The model under review builds one solid part; all positions refer to its coordinate system, in mm. Face numbers are marked on the shaded views. A direction names the side the tool comes from. Give positions to 0.01 mm unless a question says otherwise; leave off trailing zeros. Loops run counter-clockwise (first coordinate to the right, second up) from the corner with the lowest first, then second, coordinate; pieces in that order, holes last. Notation, with made-up numbers: M -6,71 L 43,71 A17 ccw 43,78 Z; hole C 76,73 d5. An arc over 180 degrees is marked long. One line per item, written item: value. Start each with the question number.
Q1. To check wall thickness, follow line 1 along X through (y, z) = (1.75, 0.5); line 2 along X through (y, z) = (1.5, 3.45); line 3 along Y through (x, z) = (-7.75, 3.6). State the ranges of each line that lie inside material, in increasing order. Write a range as from..to.
Q2. We need section A-A on y = 0. Write out the cut boundary in (x, z), plus the area to 3 significant figures.
Q3. For the marked faces 5, 6, 7, 8 and 9, list the 3-axis set-ups (+Z, -Z, +X, -X, +Y, -Y) from which the entire face can be reached by the end or side of a thin tool; tool diameter is ignored.
Q4. We need section C-C on y = 10. Write out the cut boundary in (x, z), plus the area to 3 significant figures.
Q5. Mouldability with a two-part tool opening along Y and no side actions: class the marked faces 1, 2, 3 and 4 as released by +Y, released by -Y, zero draft, split by the parting line, or undercut.
Q6. We need section B-B on x = 8.5. Write out the cut boundary in (y, z), plus the area to 3 significant figures.
Q7. For pin 1 (1.5 mm diameter, centred on x = -6, y = -8.5, fed in from +Z); pin 2 (1 mm diameter, centred on x = 1, z = 0.5, fed in from +Y), all flat-tipped, find the tip position at first contact; note any pin that passes through.
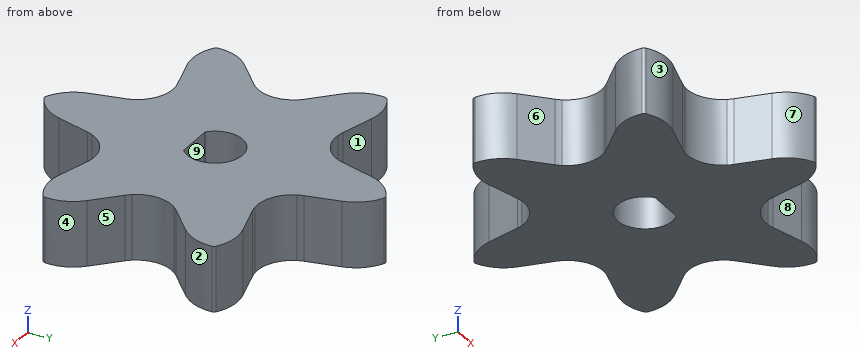
```python
from build123d import *

# Parameters (mm, degrees)
BOSS_EXTRUDE1_DEPTH = 4.7625
CUT_EXTRUDE1_DEPTH  = 4.7625


with BuildPart() as part:
    # Sketch1 → Boss-Extrude1 (new body)
    with BuildSketch(Plane.XY):
        with BuildLine():
            ThreePointArc((0.13375119, -12.340042072), (1.193950707, -11.485860744), (1.798906697, -10.266157088))
            Line((1.798906697, -10.266157088), (2.398140588, -7.862761221))
            ThreePointArc((2.398140588, -7.862761221), (2.461635419, -7.64822635), (2.543491476, -7.440004377))
            ThreePointArc((2.543491476, -7.440004377), (3.61061, -6.253759966), (5.171487057, -5.922730421))
            ThreePointArc((5.171487057, -5.922730421), (5.392740604, -5.955951983), (5.610280667, -6.008231282))
            Line((5.610280667, -6.008231282), (7.991299489, -6.690977442))
            ThreePointArc((7.991299489, -6.690977442), (9.350071835, -6.776922016), (10.619914323, -6.285852964))
            ThreePointArc((10.619914323, -6.285852964), (10.714040096, -6.185753934), (10.753665513, -6.054189108))
            ThreePointArc((10.753665513, -6.054189108), (10.544022542, -4.708938729), (9.790206185, -3.575179646))
            Line((9.790206185, -3.575179646), (8.008421255, -1.854529939))
            ThreePointArc((8.008421255, -1.854529939), (7.854376023, -1.692274367), (7.714978533, -1.517273956))
            ThreePointArc((7.714978533, -1.517273956), (7.22122, 0), (7.714978533, 1.517273956))
            ThreePointArc((7.714978533, 1.517273956), (7.854376023, 1.692274367), (8.008421255, 1.854529939))
            Line((8.008421255, 1.854529939), (9.790205754, 3.575179229))
            ThreePointArc((9.790205754, 3.575179229), (10.544022434, 4.708938449), (10.753665513, 6.054189108))
            ThreePointArc((10.753665513, 6.054189108), (10.714040096, 6.185753934), (10.619914323, 6.285852964))
            ThreePointArc((10.619914323, 6.285852964), (9.350071835, 6.776922015), (7.991299489, 6.690977442))
            Line((7.991299489, 6.690977442), (5.610280667, 6.008231282))
            ThreePointArc((5.610280667, 6.008231282), (5.392740604, 5.955951983), (5.171487057, 5.922730421))
            ThreePointArc((5.171487057, 5.922730421), (3.61061, 6.253759966), (2.543491476, 7.440004377))
            ThreePointArc((2.543491476, 7.440004377), (2.461635419, 7.64822635), (2.398140588, 7.862761221))
            Line((2.398140588, 7.862761221), (1.798906697, 10.266157088))
            ThreePointArc((1.798906697, 10.266157088), (1.193950707, 11.485860744), (0.13375119, 12.340042072))
            ThreePointArc((0.13375119, 12.340042072), (0, 12.371507867), (-0.13375119, 12.340042072))
            ThreePointArc((-0.13375119, 12.340042072), (-1.193950707, 11.485860744), (-1.798906697, 10.266157088))
            Line((-1.798906697, 10.266157088), (-2.398140588, 7.862761221))
            ThreePointArc((-2.398140588, 7.862761221), (-2.461635419, 7.64822635), (-2.543491476, 7.440004377))
            ThreePointArc((-2.543491476, 7.440004377), (-3.61061, 6.253759966), (-5.171487057, 5.922730421))
            ThreePointArc((-5.171487057, 5.922730421), (-5.392740604, 5.955951983), (-5.610280667, 6.008231282))
            Line((-5.610280667, 6.008231282), (-7.991299489, 6.690977442))
            ThreePointArc((-7.991299489, 6.690977442), (-9.350071835, 6.776922016), (-10.619914323, 6.285852964))
            ThreePointArc((-10.619914323, 6.285852964), (-10.714040096, 6.185753934), (-10.753665513, 6.054189108))
            ThreePointArc((-10.753665513, 6.054189108), (-10.544022542, 4.708938729), (-9.790206185, 3.575179646))
            Line((-9.790206185, 3.575179646), (-8.008421255, 1.854529939))
            ThreePointArc((-8.008421255, 1.854529939), (-7.854376023, 1.692274367), (-7.714978533, 1.517273956))
            ThreePointArc((-7.714978533, 1.517273956), (-7.22122, 0), (-7.714978533, -1.517273956))
            ThreePointArc((-7.714978533, -1.517273956), (-7.854376023, -1.692274367), (-8.008421255, -1.854529939))
            Line((-8.008421255, -1.854529939), (-9.790205754, -3.575179229))
            ThreePointArc((-9.790205754, -3.575179229), (-10.544022434, -4.708938449), (-10.753665513, -6.054189108))
            ThreePointArc((-10.753665513, -6.054189108), (-10.714040096, -6.185753934), (-10.619914323, -6.285852964))
            ThreePointArc((-10.619914323, -6.285852964), (-9.350071835, -6.776922015), (-7.991299489, -6.690977442))
            Line((-7.991299489, -6.690977442), (-5.610280667, -6.008231282))
            ThreePointArc((-5.610280667, -6.008231282), (-5.392740604, -5.955951983), (-5.171487057, -5.922730421))
            ThreePointArc((-5.171487057, -5.922730421), (-3.61061, -6.253759966), (-2.543491476, -7.440004377))
            ThreePointArc((-2.543491476, -7.440004377), (-2.461635419, -7.64822635), (-2.398140588, -7.862761221))
            Line((-2.398140588, -7.862761221), (-1.798906697, -10.266157088))
            ThreePointArc((-1.798906697, -10.266157088), (-1.193950707, -11.485860744), (-0.13375119, -12.340042072))
            ThreePointArc((-0.13375119, -12.340042072), (0, -12.371507867), (0.13375119, -12.340042072))
        make_face()
        with BuildLine():
            Line((1.313392554, -1.475), (-1.313392554, -1.475))
            ThreePointArc((-1.313392554, -1.475), (0, 1.975), (1.313392554, -1.475))
        make_face(mode=Mode.SUBTRACT)
    extrude(amount=BOSS_EXTRUDE1_DEPTH)

    # Sketch2 → Cut-Extrude1 (cut)
    with BuildSketch(Plane.XY.offset(4.7625)):
        with BuildLine():
            Line((-1.322875656, -1.5), (1.322875656, -1.5))
            ThreePointArc((1.322875656, -1.5), (0, 2), (-1.322875656, -1.5))
        make_face()
    extrude(amount=-CUT_EXTRUDE1_DEPTH, mode=Mode.SUBTRACT)


solid = part.part
```
Solved:
1. line 1: -7.91..-0.97, 0.97..7.91
1. line 2: -7.7..-1.32, 1.32..7.7
1. line 3: -6.62..-1.56, 1.56..6.62
2. outline: M -7.22,0 L -2,0 L -2,4.76 L -7.22,4.76 Z; M 2,0 L 7.22,0 L 7.22,4.76 L 2,4.76 Z
2. area: 49.7 mm2
3. face 5: +Z, -Z, +X
3. face 6: +Z, -Z, -X
3. face 7: +Z, -Z, -X, -Y
3. face 8: +Z, -Z, -Y
3. face 9: +Z, -Z
4. outline: M -1.87,0 L 1.87,0 L 1.87,4.76 L -1.87,4.76 Z
4. area: 17.8 mm2
5. face 1: released by +Y
5. face 2: undercut
5. face 3: released by -Y
5. face 4: undercut
6. outline: M -6.79,0 L -2.33,0 L -2.33,4.76 L -6.79,4.76 Z; M 2.33,0 L 6.79,0 L 6.79,4.76 L 2.33,4.76 Z
6. area: 42.5 mm2
7. pin 1: through
7. pin 2: y = 12.13
